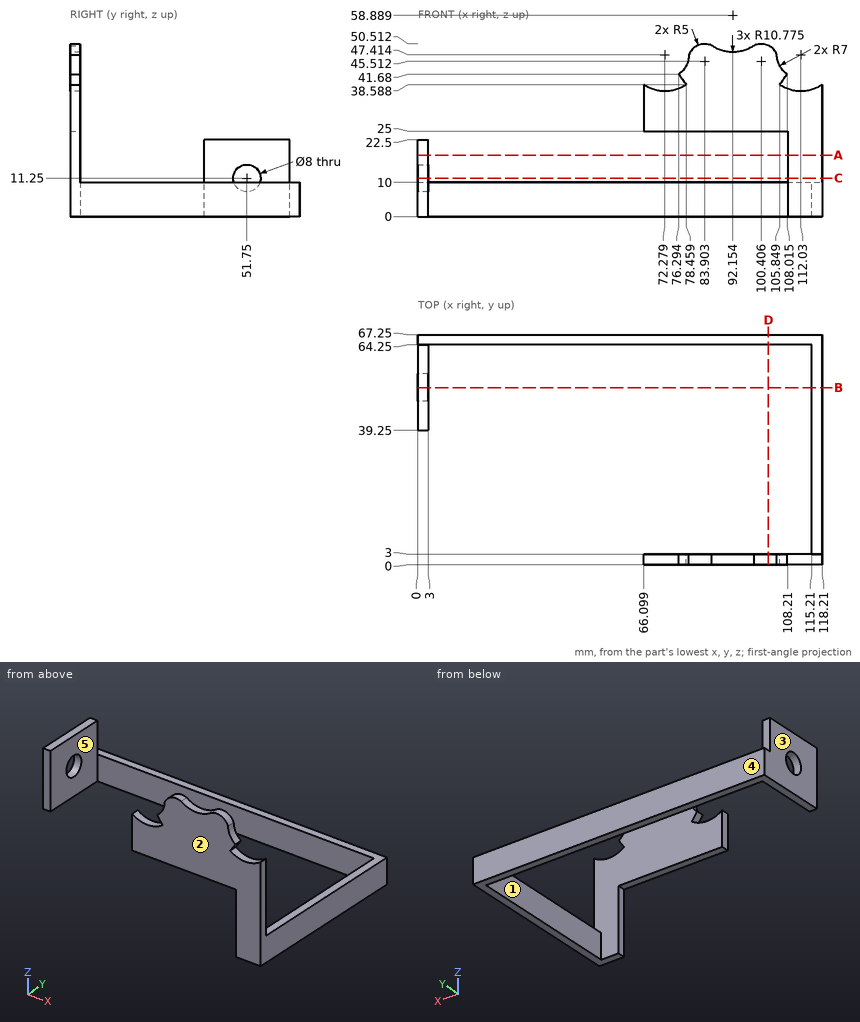
Check sheet for the drawn part. Datum: minimum x, y, z corner. Units: mm. A direction names the side the tool comes from. Round coordinates to 2 decimals unless told otherwise and drop trailing zeros. Order: outer loops, then holes, each group sorted by start corner. A loop starts at its lowest first (then second) coordinate and runs counter-clockwise, first axis right, second up. Notation, with made-up numbers: (19, 37) - (60, 37) arc R15 ccw to (60, 42) - close; hole circle Ø3 at (-0.5, -20.5). An arc over 180 degrees is marked (long way). Use a Markdown table: item, result. Add a question column.
(1) Depth check by flat-ended pin: pin 1 (1.5 mm diameter, centred on x = 2, z = 12, fed in from -Y); pin 2 (0.9 mm diameter, centred on x = 96.5, y = 2, fed in from -Z); pin 3 (0.9 mm diameter, centred on y = 1, z = 9.5, fed in from -X). Enter the tip coordinate at first touch or a pass-through.
(2) Release check for a two-part mould opening along Y. For the marked faces 1, 2 and 3 record: pulls with the +Y half, pulls with the -Y half, needs draft (parallel to the pull), parting line crosses it, or undercut.
(3) Sectioned sample at B-B, the plane y = 51.75. Enter the section's corners in (x, z).
(4) Tool access check on the marked faces 4 and 5. Record the directions out of +Z, -Z, +X, -X, +Y, -Y that give a thin tool (end or side, any length) a straight path to the whole face; none if there is none.
(5) Material ranges on line 1 along Y through (x, z) = (1, 11); line 2 along X through (y, z) = (62, 3); line 3 along Y through (x, z) = (51.5, 9), recorded low to high. Write a range as [from, to].
(6) Sectioned sample at A-A, the plane z = 18. Enter the section's corners in (x, y), and give its area (3 significant figures).
(7) Sectioned sample at D-D, the plane x = 102.5. Enter the section's corners in (y, z), and give its area (3 significant figures).
(8) Sectioned sample at C-C, the plane z = 11.25. Enter the section's corners in (x, y).
Answers below:
| question | item | result |
|---|---|---|
| 1 | pin 1 | y = 39.25 |
| 1 | pin 2 | z = 25 |
| 1 | pin 3 | x = 108.21 |
| 2 | face 1 | undercut |
| 2 | face 2 | pulls with the -Y half |
| 2 | face 3 | needs draft |
| 3 | outline | (0, 0) - (3, 0) - (3, 7.25) - (0, 7.25) - close; (0, 15.25) - (3, 15.25) - (3, 22.5) - (0, 22.5) - close; (115.21, 0) - (118.21, 0) - (118.21, 10) - (115.21, 10) - close |
| 4 | face 4 | +Z, -Z, +X, -X, +Y |
| 4 | face 5 | +Z, -Z, -Y |
| 5 | line 1 | [39.25, 47.76], [55.74, 64.25] |
| 5 | line 2 | [0, 3], [115.21, 118.21] |
| 5 | line 3 | [64.25, 67.25] |
| 6 | outline | (0, 39.25) - (3, 39.25) - (3, 64.25) - (0, 64.25) - close; (108.21, 0) - (118.21, 0) - (118.21, 3) - (108.21, 3) - close |
| 6 | area | 105 mm² |
| 7 | outline | (0, 25) - (3, 25) - (3, 50.05) - (0, 50.05) - close; (64.25, 0) - (67.25, 0) - (67.25, 10) - (64.25, 10) - close |
| 7 | area | 105 mm² |
| 8 | outline | (0, 39.25) - (3, 39.25) - (3, 47.75) - (0, 47.75) - close; (0, 55.75) - (3, 55.75) - (3, 64.25) - (0, 64.25) - close; (108.21, 0) - (118.21, 0) - (118.21, 3) - (108.21, 3) - close |
